Model file for the job. Use its own axes, mm. Round coordinates to 2 decimals unless told otherwise and drop trailing zeros. Order: outer loops, then holes, each group sorted by start corner. A loop starts at its lowest first (then second) coordinate and runs counter-clockwise, first axis right, second up. Notation, with made-up numbers: (76.25, 81.25) - (88.25, 81.25) arc R22 cw to (88.25, 114.25) - close; hole circle Ø9 at (11.25, 45). An arc over 180 degrees is marked (long way). Put each result on its own line as item: value. Start each with the question number.
Item 1: Saw through at C-C on x = 0. List the corners of the cut face in (y, z), plus the area to 3 significant figures.
Item 2: Saw through at B-B on z = 2.15. List the corners of the cut face in (x, y).
Item 3: Saw through at A-A on y = 0. List the corners of the cut face in (x, z), plus the area to 3 significant figures.
Item 4: Mould opens along Y. For faces 1 (the face through (-1, 3, 3)), 2 (the face through (-1, -6, 1)), 3 (the face through (-0.54, 2.44, 1.48)) say: pulls with the +Y half, pulls with the -Y half, needs draft (parallel to the pull), parting line crosses it, or undercut.
Item 5: Probe probe 1 along Y at (x, z) = (0, 1.45); probe 2 along X at (y, z) = (-1, 2.25); probe 3 along X at (y, z) = (-1.5, 2.45). List the from-to ranges inside material, lowest first.
Autodesk Inventor part; units mm, degrees
ref_plane "YZ Plane" through (0, 0, 0) normal (1, 0, 0) x (0, 1, 0)
ref_plane "XZ Plane" through (0, 0, 0) normal (0, 1, 0) x (-1, 0, 0)
ref_plane "XY Plane" through (0, 0, 0) normal (0, 0, 1) x (1, 0, 0)
sketch "草圖1" plane through (0, 0, 0) normal (0, 0, 1) x (1, 0, 0)
  line L0 (-60.5, 0) -> (60.5, 0) construction
  line L1 (-60.5, -6) -> (60.5, -6)
  line L2 (60.5, 6) -> (-60.5, 6)
  arc A0 (-60.5, 6) -> (-60.5, -6) centre (-60.5, 0) ccw
  arc A1 (60.5, -6) -> (60.5, 6) centre (60.5, 0) ccw
  circle A2 centre (-60.5, 0) radius 2.5
  circle A3 centre (0, 0) radius 2.5
  circle A4 centre (60.5, 0) radius 2.5
  dimension "d0" = 121
  dimension "d1" = 12
  dimension "d2" = 5
extrude "擠出1" add sketch "草圖1" along normal blind 3
sketch "草圖2" plane through (0, 0, 3) normal (0, 0, 1) x (1, 0, 0)
  arc A0 (60.5, -6) -> (60.5, 6) centre (60.5, 0) ccw
  line L0 (60.5, 6) -> (-60.5, 6)
  arc A1 (-60.5, 6) -> (-60.5, -6) centre (-60.5, 0) ccw
  line L1 (-60.5, -6) -> (60.5, -6)
  circle A2 centre (0, 0) radius 2.5
  circle A3 centre (60.5, 0) radius 2.5
  circle A4 centre (-60.5, 0) radius 2.5
properties part number "連桿"
Results found:
1. outline: (-6, 0) - (-2.5, 0) - (-2.5, 3) - (-6, 3) - close; (2.5, 0) - (6, 0) - (6, 3) - (2.5, 3) - close
1. area: 21.0 mm²
2. outline: (-60.5, -6) - (60.5, -6) arc R6 ccw to (60.5, 6) - (-60.5, 6) arc R6 ccw to start; hole circle Ø5 at (-60.5, 0); hole circle Ø5 at (0, 0); hole circle Ø5 at (60.5, 0)
3. outline: (-66.5, 0) - (-63, 0) - (-63, 3) - (-66.5, 3) - close; (-58, 0) - (-2.5, 0) - (-2.5, 3) - (-58, 3) - close; (2.5, 0) - (58, 0) - (58, 3) - (2.5, 3) - close; (63, 0) - (66.5, 0) - (66.5, 3) - (63, 3) - close
3. area: 354 mm²
4. face 1: needs draft
4. face 2: pulls with the -Y half
4. face 3: undercut
5. probe 1: y = -6 to -2.5, 2.5 to 6
5. probe 2: x = -66.42 to -62.79, -58.21 to -2.29, 2.29 to 58.21, 62.79 to 66.42
5. probe 3: x = -66.31 to -62.5, -58.5 to -2, 2 to 58.5, 62.5 to 66.31
